Verification items for the finished model (mm, model axes). Face numbers are marked on the shaded views. A direction names the side the tool comes from. Round coordinates to 2 decimals unless told otherwise and drop trailing zeros. Order: outer loops, then holes, each group sorted by start corner. A loop starts at its lowest first (then second) coordinate and runs counter-clockwise, first axis right, second up. Notation, with made-up numbers: (-39.5, -21.5) -> (-1.5, -21.5) arc R7 cw to (-1.5, -16.5) -> close; hole circle Ø9 at (-9, -20.75). An arc over 180 degrees is marked (long way). Put each result on its own line as item: value.
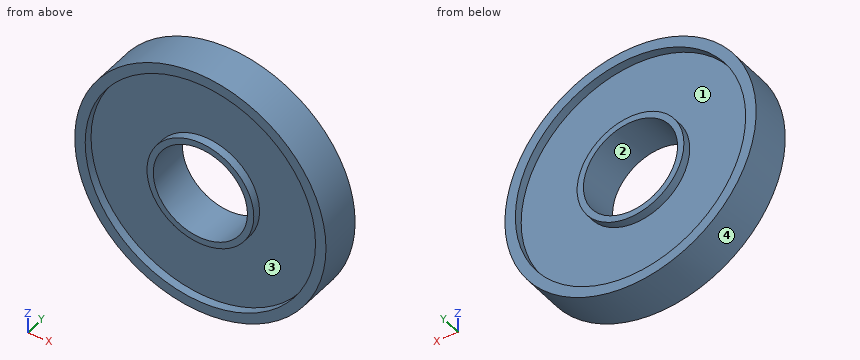
from build123d import *

# Parameters (mm, degrees)
F0_R      = 30
F1_DEPTH  = 10
F2_R      = 27.5
F3_DEPTH  = 2
F4_R      = 27.5
F5_DEPTH  = 2
F6_R      = 12.75
F7_DEPTH  = 2
F8_R      = 12.75
F9_DEPTH  = 2
F10_R     = 11.25
F11_DEPTH = 10.001


with BuildPart() as f1:
    # F0 (on Front) → F1 (new body)
    with BuildSketch(Plane.XZ):
        with Locations((-21.965394, 3.416839)):
            Circle(F0_R)
    extrude(amount=F1_DEPTH)

    # F2 (on face) → F3 (cut)
    with BuildSketch(Plane.XZ.offset(10)):
        with Locations((-21.965394, 3.416839)):
            Circle(F2_R)
    extrude(amount=-F3_DEPTH, mode=Mode.SUBTRACT)

    # F4 (on face) → F5 (cut)
    with BuildSketch(Plane(origin=(0, 0, 0), x_dir=(-1, 0, 0), z_dir=(0, 1, 0))):
        with Locations((21.965394, 3.416839)):
            Circle(F4_R)
    extrude(amount=-F5_DEPTH, mode=Mode.SUBTRACT)

    # F6 (on face) → F7 (join)
    with BuildSketch(Plane(origin=(0, -2, 0), x_dir=(-1, 0, 0), z_dir=(0, 1, 0))):
        with Locations((21.965394, 3.416839)):
            Circle(F6_R)
    extrude(amount=F7_DEPTH)

    # F8 (on face) → F9 (join)
    with BuildSketch(Plane.XZ.offset(8)):
        with Locations((-21.965394, 3.416839)):
            Circle(F8_R)
    extrude(amount=F9_DEPTH)

    # F10 (on face) → F11 (cut, through all)
    with BuildSketch(Plane.XZ.offset(10)):
        with Locations((-21.965394, 3.416839)):
            Circle(F10_R)
    extrude(amount=-F11_DEPTH, mode=Mode.SUBTRACT)


solid = f1.part
Item 1: Tool access check on the marked faces 1 and 2. Record the directions out of +Z, -Z, +X, -X, +Y, -Y that give a thin tool (end or side, any length) a straight path to the whole face; none if there is none.
Check sheet entries:
face 1: +Y
face 2: +Y, -Y
Item 2: Section check B-B on x = -32. Record the boundary of the cut face in (y, z).
Check sheet entries:
outline: (-10, -24.86) -> (0, -24.86) -> (0, -22.19) -> (-2, -22.19) -> (-2, -4.45) -> (0, -4.45) -> (0, -1.67) -> (-10, -1.67) -> (-10, -4.45) -> (-8, -4.45) -> (-8, -22.19) -> (-10, -22.19) -> close; (-10, 8.5) -> (0, 8.5) -> (0, 11.28) -> (-2, 11.28) -> (-2, 29.02) -> (0, 29.02) -> (0, 31.69) -> (-10, 31.69) -> (-10, 29.02) -> (-8, 29.02) -> (-8, 11.28) -> (-10, 11.28) -> close
Item 3: Gauge pin test, flat ends, axial feed: pin 1 Ø1 at (y, z) = (-7.5, -9.5) entering from +X; pin 2 Ø3 at (x, y) = (-3, -7) entering from +Z; pin 3 Ø5 at (y, z) = (-2.5, -14.5) entering from -X. Record the tip position at first contact, or that the pin passes through.
Check sheet entries:
pin 1: stops at x = 5.34
pin 2: stops at z = 27.81
pin 3: stops at x = -47.7
Item 4: Section check A-A on z = -6. Record the boundary of the cut face in (x, y).
Check sheet entries:
outline: (-50.45, -10) -> (-47.8, -10) -> (-47.8, -8) -> (-30.56, -8) -> (-30.56, -10) -> (-28.12, -10) -> (-28.12, 0) -> (-30.56, 0) -> (-30.56, -2) -> (-47.8, -2) -> (-47.8, 0) -> (-50.45, 0) -> close; (-15.81, -10) -> (-13.37, -10) -> (-13.37, -8) -> (3.87, -8) -> (3.87, -10) -> (6.52, -10) -> (6.52, 0) -> (3.87, 0) -> (3.87, -2) -> (-13.37, -2) -> (-13.37, 0) -> (-15.81, 0) -> close
Item 5: Release check for a two-part mould opening along Z. For the marked faces 3 and 4 record: +Z half, -Z half, draft (parallel to the pull), parting line (faces both ways), or undercut.
Check sheet entries:
face 3: undercut
face 4: parting line
Item 6: Section check C-C on y = -1.25. Record the boundary of the cut face in (x, z).
Check sheet entries:
outline: circle Ø60 at (-21.97, 3.42); circle Ø25.5 at (-21.97, 3.42); hole circle Ø55 at (-21.97, 3.42); hole circle Ø22.5 at (-21.97, 3.42)
Item 7: Section check D-D on x = -4.5. Record the boundary of the cut face in (y, z), then the cut area to 3 significant figures.
Check sheet entries:
outline: (-10, -20.97) -> (0, -20.97) -> (0, -17.82) -> (-2, -17.82) -> (-2, 24.66) -> (0, 24.66) -> (0, 27.81) -> (-10, 27.81) -> (-10, 24.66) -> (-8, 24.66) -> (-8, -17.82) -> (-10, -17.82) -> close
area: 318 mm^2
Item 8: Material ranges on L1, parallel to X at y = -8.5, z = 4; L2, parallel to Z at x = -26, y = -1; L3, parallel to Z at x = -12, y = -1.5, recorded low to high. Write a range as [from, to].
Check sheet entries:
L1: x = [-51.96, -49.46], [-34.7, -33.2], [-10.73, -9.23], [5.53, 8.03]
L2: z = [-26.31, -23.79], [-8.68, -7.08], [13.92, 15.51], [30.62, 33.14]
L3: z = [-24.88, -22.21], [-4.54, -1.8], [8.64, 11.37], [29.05, 31.71]
